from build123d import *

# Parameters (mm, degrees)
EXTRUDE_THIN1_DEPTH = 285.75
FILLET1_R           = 1.27


with BuildPart() as part:
    # Sketch1 → Extrude-Thin1 (new body)
    with BuildSketch(Plane.XY):
        Polygon((-14.2875, 0), (-14.2875, 4.7625), (-4.7625, 4.7625), (-4.7625, 1.666875), (4.7625, 1.666875), (4.7625, 4.7625), (14.2875, 4.7625), (14.2875, 0), (13.0175, 0), (13.0175, 3.4925), (6.0325, 3.4925), (6.0325, 0.396875), (-6.0325, 0.396875), (-6.0325, 3.4925), (-13.0175, 3.4925), (-13.0175, 0), align=None)
    extrude(amount=-EXTRUDE_THIN1_DEPTH)

    # Fillet1
    fillet1_edges = [part.edges().sort_by_distance(p)[0] for p in [
        (-14.2875, 4.7625, -142.875),
        (-4.7625, 4.7625, -142.875),
        (4.7625, 4.7625, -142.875),
        (14.2875, 4.7625, -142.875),
        (6.0325, 0.396875, -142.875),
        (-6.0325, 0.396875, -142.875),
    ]]
    fillet(fillet1_edges, radius=FILLET1_R)


solid = part.part
Design review of the part built by this model. Coordinates are the model's own, in mm. A direction names the side the tool comes from. Coordinates: 2 decimals unless noted, no trailing zeros. Order: outer loops, then holes, each group sorted by start corner. A loop starts at its lowest first (then second) coordinate and runs counter-clockwise, first axis right, second up. Notation, with made-up numbers: (19, 58.5) -> (74, 58.5) arc R30 ccw to (74, 90.5) -> close; hole circle Ø9 at (53.25, 74.25). An arc over 180 degrees is marked (long way). Use one line per item in the form item = value. Start each with the question number.
(1) Insertion check: pin 1 (2 mm diameter, centred on x = 8.5, z = -149.5, fed in from -Y); pin 2 (5 mm diameter, centred on x = -0.5, z = -122, fed in from +Y); pin 3 (3 mm diameter, centred on x = 2, z = -79.5, fed in from -Y). Each pin has a flat end and moves straight along its axis. Give the tip position at first contact, or say it passes through.
(2) For probe 1 along X at (y, z) = (2.6, -34); probe 2 along Y at (x, z) = (-11.25, -33.5); probe 3 along Y at (x, z) = (-4, -23), list the stretches that pass through material, from the lowest coordinate up.
(3) Add section A-A on z = -85.5. State the section outline as (x, y) points.
(4) Add section B-B on x = 1. State the section outline as (y, z) points.
(5) For faces 1 (the flat face through (-9, 3.492, -141)), 2 (the flat face through (0, 1, 0)), list the 3-axis set-ups (+Z, -Z, +X, -X, +Y, -Y) from which the entire face can be reached by the end or side of a thin tool; tool diameter is ignored.
(6) The part is to be moulded in two halves that separate along X. For faces 3 (the flat face through (0, 1.667, -141)), 4 (the flat face through (-10, 4.762, -141)), say which applies: +X half, -X half, draft (parallel to the pull), parting line (faces both ways), or undercut.
Answer block:
q1.pin_1 = 3.49
q1.pin_2 = 1.67
q1.pin_3 = 0.4
q2.probe_1 = -14.29 to -13.02, -6.03 to -4.76, 4.76 to 6.03, 13.02 to 14.29
q2.probe_2 = 3.49 to 4.76
q2.probe_3 = 0.4 to 1.67
q3.outline = (-14.29, 0) -> (-13.02, 0) -> (-13.02, 3.49) -> (-6.03, 3.49) -> (-6.03, 1.67) arc R1.27 ccw to (-4.76, 0.4) -> (4.76, 0.4) arc R1.27 ccw to (6.03, 1.67) -> (6.03, 3.49) -> (13.02, 3.49) -> (13.02, 0) -> (14.29, 0) -> (14.29, 3.49) arc R1.27 ccw to (13.02, 4.76) -> (6.03, 4.76) arc R1.27 ccw to (4.76, 3.49) -> (4.76, 1.67) -> (-4.76, 1.67) -> (-4.76, 3.49) arc R1.27 ccw to (-6.03, 4.76) -> (-13.02, 4.76) arc R1.27 ccw to (-14.29, 3.49) -> close
q4.outline = (0.4, -285.75) -> (1.67, -285.75) -> (1.67, 0) -> (0.4, 0) -> close
q5.face_1 = +Z, -Z, -Y
q5.face_2 = +Z, +X, -X, +Y, -Y
q6.face_3 = undercut
q6.face_4 = draft
